Could you check a few things on this model? Use its own coordinates, in mm. Face numbers are marked on the shaded views. A direction names the side the tool comes from. Round coordinates to 2 decimals unless told otherwise and drop trailing zeros. Order: outer loops, then holes, each group sorted by start corner. A loop starts at its lowest first (then second) coordinate and runs counter-clockwise, first axis right, second up. Notation, with made-up numbers: M -32,73.25 L 10,73.25 A21 cw 10,97.25 Z; hole C -1.5,36.5 d11. An arc over 180 degrees is marked long. Write each question's results on one line, items separated by ' | '. Start each with the question number.
1. Please list where these lines run through material, in increasing order: L1, parallel to Y at x = 11, z = 23.25; L2, parallel to X at y = 3, z = 9; L3, parallel to Z at x = 9, y = -1.
2. We'd pull the mould along X, two halves only. Please class the marked faces 1, 2 and 3: released by +X, released by -X, zero draft, split by the parting line, or undercut.
3. Suppose I cut it at B-B on x = 5. Write out the boundary of the cut face in (y, z), and give its area (3 significant figures).
4. Suppose I cut it at D-D on x = -23. Write out the boundary of the cut face in (y, z), and give its area (3 significant figures).
5. Suppose I cut it at A-A on y = 0. Write out the boundary of the cut face in (x, z).
6. For the marked faces 4, 5 and 6, which set-ups out of +Z, -Z, +X, -X, +Y, -Y let a thin tool reach every point of the face, with its end or its side?
7. I'm going to push flat-ended pins straight in: pin 1 (2 mm diameter, centred on y = 4, z = 10.5, fed in from +X); pin 2 (3.5 mm diameter, centred on y = -0.5, z = 10.5, fed in from +X); pin 3 (2.5 mm diameter, centred on x = 9, z = 18.5, fed in from +Y). Where does each tip first touch, or does it pass through?
8. Suppose I cut it at C-C on z = 15. Write out the boundary of the cut face in (x, y).
from build123d import *

# Parameters (mm, degrees)
F1_DEPTH       = 25
F2_W           = 10
F2_H           = 19
F3_DEPTH       = 3
F4_R           = 9
F5_DEPTH       = 10
F6_R           = 2.5
F7_DEPTH       = 25
F8_W           = 3
F8_H           = 6
F9_DEPTH       = 6
F10_R          = 1
F11_DEPTH      = 25
F13_DEPTH      = 25
F13_DEPTH_BACK = 2


with BuildPart() as f1:
    # F0 (on Top) → F1 (new body)
    with BuildSketch(Plane.XY):
        Polygon((1.6985263115, 0.4360290599), (1.6985263115, 2.7860290599), (11.6985263115, 2.7860290599), (11.6985263115, 5.7860290599), (-2.3014736885, 5.7860290599), (-2.3014736885, 2.4360290599), (-27.3014736885, 2.4360290599), (-27.3014736885, -2.5639709401), (11.6985263115, -2.5639709401), (11.6985263115, 0.4360290599), align=None)
    extrude(amount=F1_DEPTH)

    # F2 (on face) → F3 (cut)
    with BuildSketch(Plane(origin=(0, 5.7860290599, 0), x_dir=(-1, 0, 0), z_dir=(0, 1, 0))):
        with Locations((-6.6985263115, 15.5)):
            Rectangle(F2_W, F2_H)
    extrude(amount=-F3_DEPTH, mode=Mode.SUBTRACT)

    # F4 (on face) → F5 (cut)
    with BuildSketch(Plane(origin=(0, 2.4360290599, 0), x_dir=(-1, 0, 0), z_dir=(0, 1, 0))):
        with Locations((14.8014736885, 12.5)):
            Circle(F4_R)
    extrude(amount=-F5_DEPTH, mode=Mode.SUBTRACT)

    # F6 (on face) → F7 (cut)
    with BuildSketch(Plane(origin=(0, 0.4360290599, 0), x_dir=(-1, 0, 0), z_dir=(0, 1, 0))):
        with Locations((-6.8985263115, 15)):
            Circle(F6_R)
    extrude(amount=-F7_DEPTH, mode=Mode.SUBTRACT)

    # F8 (on face) → F9 (join)
    with BuildSketch(Plane.YZ.offset(11.6985263115)):
        with Locations((4.2860290599, 3)):
            Rectangle(F8_W, F8_H)
    extrude(amount=F9_DEPTH)

    # F10 (on face) → F11 (cut)
    with BuildSketch(Plane.XY.offset(25)):
        with Locations((1.6985263115, 0.4360290599)):
            Circle(F10_R)
    extrude(amount=-F11_DEPTH, mode=Mode.SUBTRACT)

    # F12 (on face) → F13 (cut, two sides)
    with BuildSketch(Plane.XY.offset(6)) as f13_sk:
        with BuildLine():
            ThreePointArc((1.6985263115, 3.7860290599), (0.9914195303, 2.0789222787), (2.6985263115, 2.7860290599))
            Line((2.6985263115, 2.7860290599), (1.6985263115, 2.7860290599))
            Line((1.6985263115, 2.7860290599), (1.6985263115, 3.7860290599))
        make_face()
        with BuildLine():
            Line((1.6985263115, 2.7860290599), (2.6985263115, 2.7860290599))
            ThreePointArc((2.6985263115, 2.7860290599), (2.4056330927, 3.4931358411), (1.6985263115, 3.7860290599))
            Line((1.6985263115, 3.7860290599), (1.6985263115, 2.7860290599))
        make_face()
    extrude(amount=-F13_DEPTH, mode=Mode.SUBTRACT)
    extrude(f13_sk.sketch, amount=F13_DEPTH_BACK, mode=Mode.SUBTRACT)


solid = f1.part
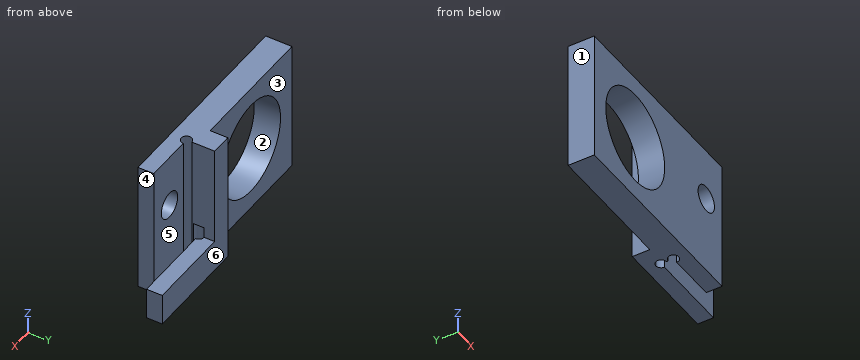
Filled sheet:
1) L1: y = -2.56 to 0.44 | L2: x = -2.3 to 1.7 | L3: z = 0 to 13.65, 16.35 to 25
2) face 1: released by -X | face 2: undercut | face 3: zero draft
3) outline: M -2.56,0 L 0.44,0 L 0.44,13.37 L -2.56,13.37 Z; M -2.56,16.63 L 0.44,16.63 L 0.44,25 L -2.56,25 Z; M 2.79,0 L 5.79,0 L 5.79,6 L 2.79,6 Z | area: 83.2 mm^2
4) outline: M -2.56,0 L 2.44,0 L 2.44,8.79 L -2.56,8.79 Z; M -2.56,16.21 L 2.44,16.21 L 2.44,25 L -2.56,25 Z | area: 87.9 mm^2
5) outline: M -27.3,0 L 0.8,0 L 0.8,25 L -27.3,25 Z; M 2.6,0 L 11.7,0 L 11.7,25 L 2.6,25 Z; hole C -14.8,12.5 d18; hole C 6.9,15 d5
6) face 4: +Z, -Z, +X, -Y | face 5: +Z, -Z, +X | face 6: +Z, -Z, +X, -X, +Y
7) pin 1: stops at x = 1.7 | pin 2: stops at x = 11.7 | pin 3: stops at y = 0.44
8) outline: M -27.3,-2.56 L -23.45,-2.56 L -23.45,2.44 L -27.3,2.44 Z; M -6.16,-2.56 L 4.4,-2.56 L 4.4,0.44 L 2.7,0.44 A1 cw long 1.7,1.44 L 1.7,5.79 L -2.3,5.79 L -2.3,2.44 L -6.16,2.44 Z; M 9.4,-2.56 L 11.7,-2.56 L 11.7,0.44 L 9.4,0.44 Z
